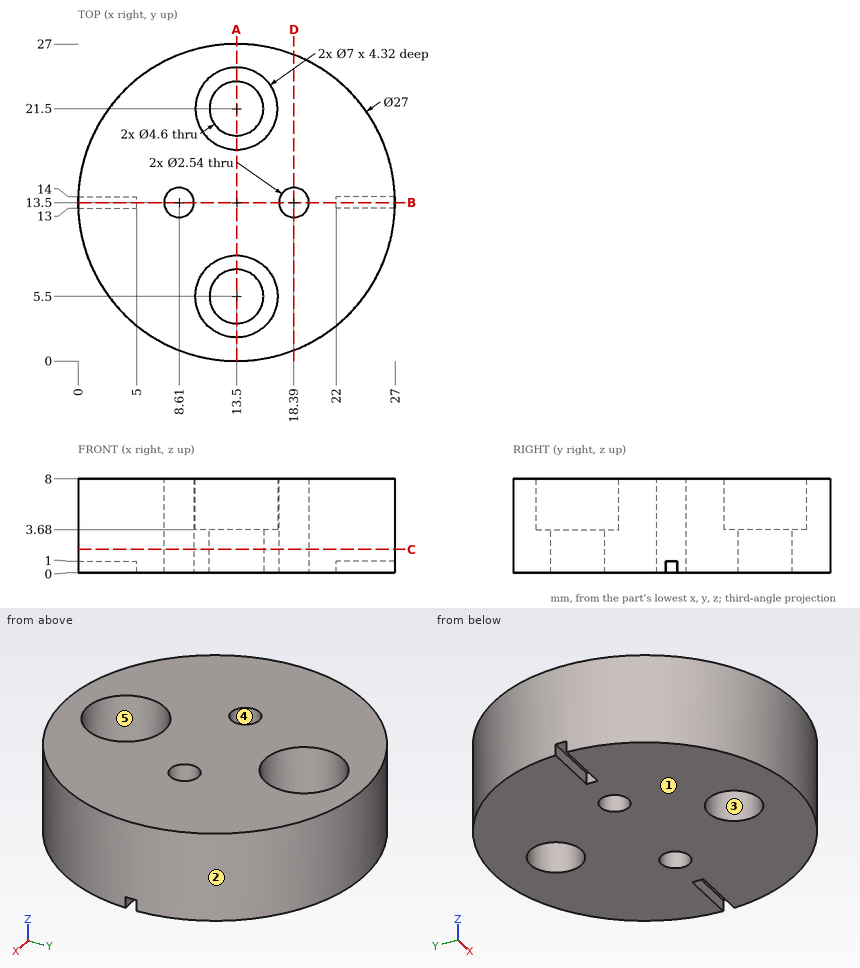
Study the drawing (mm; zero at the part's minimum x, y, z) and answer. A direction names the side the tool comes from. Coordinates: 2 decimals unless noted, no trailing zeros. Write each loop counter-clockwise with the first axis right and the second up, starting at its lowest first coordinate (ties: lowest second). Pieces come first, ordered by that corner, then holes. Notation, with made-up numbers: (61, 58.25) - (108, 58.25) arc R16 ccw to (108, 67.25) - close; hole circle Ø10 at (46.25, 48.5). An arc over 180 degrees is marked (long way). Put each result on its own line as item: value.
1. Find the intervals of material crossed by line 1 along Y through (x, z) = (12.5, 6.75); line 2 along Y through (x, z) = (18.39, 3); line 3 along Y through (x, z) = (17.75, 3.5), in increasing order. Write a range as from..to.
Answer sheet:
line 1: y = 0.04..2.15, 8.85..18.15, 24.85..26.96
line 2: y = 0.92..12.23, 14.77..26.08
line 3: y = 0.69..12.4, 14.6..26.31
2. The part is cut by section B-B on y = 13.5. Give the vertices of the cut face in (x, z).
Answer sheet:
outline: (0, 1) - (5, 1) - (5, 0) - (7.34, 0) - (7.34, 8) - (0, 8) - close; (9.88, 0) - (17.12, 0) - (17.12, 8) - (9.88, 8) - close; (19.66, 0) - (22, 0) - (22, 1) - (27, 1) - (27, 8) - (19.66, 8) - close
3. Determine the mould class of the marked faces 1, 2 and 3 for opening direction Y: pulls with the +Y half, pulls with the -Y half, needs draft (parallel to the pull), parting line crosses it, or undercut.
Answer sheet:
face 1: needs draft
face 2: parting line crosses it
face 3: undercut
4. The part is cut by section C-C on z = 2. Give the vertices of the cut face in (x, y), plus the area to 3 significant figures.
Answer sheet:
outline: circle Ø27 at (13.5, 13.5); hole circle Ø2.54 at (8.61, 13.5); hole circle Ø4.6 at (13.5, 5.5); hole circle Ø4.6 at (13.5, 21.5); hole circle Ø2.54 at (18.39, 13.5)
area: 529 mm^2
5. The part is cut by section A-A on x = 13.5. Give the vertices of the cut face in (y, z), plus the area to 3 significant figures.
Answer sheet:
outline: (0, 0) - (3.2, 0) - (3.2, 3.68) - (2, 3.68) - (2, 8) - (0, 8) - close; (7.8, 0) - (19.2, 0) - (19.2, 3.68) - (18, 3.68) - (18, 8) - (9, 8) - (9, 3.68) - (7.8, 3.68) - close; (23.8, 0) - (27, 0) - (27, 8) - (25, 8) - (25, 3.68) - (23.8, 3.68) - close
area: 122 mm^2
6. Flat-ended cylindrical pins translate along their axes: pin 1 Ø1.1 at (y, z) = (13.5, 0.5) entering from -X; pin 2 Ø1 at (x, z) = (18.5, 5.5) entering from +Y; pin 3 Ø3 at (x, y) = (13, 5.5) entering from -Z; pin 4 Ø0.8 at (y, z) = (13.5, 0.5) entering from +X. Find the tip coordinate at first contact, or state that the pin passes through.
Answer sheet:
pin 1: stops at x = 0
pin 2: stops at y = 26.23
pin 3: passes through
pin 4: stops at x = 22
7. A tool of negligible diameter and unlimited length cuts with its end or side. For the marked faces 4 and 5, from which of +Z, -Z, +X, -X, +Y, -Y can it reach the whole face along a straight path? Write none if from no direction.
Answer sheet:
face 4: +Z, -Z
face 5: +Z
8. The part is cut by section D-D on x = 18.39. Give the vertices of the cut face in (y, z), plus the area to 3 significant figures.
Answer sheet:
outline: (0.92, 0) - (12.23, 0) - (12.23, 8) - (0.92, 8) - close; (14.77, 0) - (26.08, 0) - (26.08, 8) - (14.77, 8) - close
area: 181 mm^2
